```python
from build123d import *

# Parameters (mm, degrees)
PAD_DEPTH       = 35
SKETCH001_W     = 64.566103
SKETCH001_H     = 15
POCKET_DEPTH    = 35
PAD001_DEPTH    = 2
FILLET_R        = 1
FILLET001_R     = 1
FILLET002_R     = 1
FILLET003_R     = 1
FILLET004_R     = 1
PAD002_DEPTH    = 2
FILLET005_R     = 1
FILLET006_R     = 1
FILLET007_R     = 0.8
SKETCH005_R     = 1.8
POCKET001_DEPTH = 5
CHAMFER_SIZE    = 1
CHAMFER001_SIZE = 1
SKETCH006_W     = 10.45074
SKETCH006_H     = 39.185364
POCKET002_DEPTH = 5
SKETCH007_W     = 9.636787
SKETCH007_H     = 41.557176
POCKET003_DEPTH = 5
FILLET008_R     = 10
FILLET009_R     = 10


with BuildPart() as part:
    # Sketch → Pad (new body)
    with BuildSketch(Plane.XY):
        with BuildLine():
            ThreePointArc((25, 0), (0, 25), (-25, 0))
            Line((-27, 0), (-25, 0))
            ThreePointArc((27, 0), (0, 27), (-27, 0))
            Line((27, 0), (25, 0))
        make_face()
    extrude(amount=PAD_DEPTH)

    # Sketch001 (on Face6 of Pad) → Pocket (cut)
    with BuildSketch(Plane.XY.offset(35)):
        with Locations((1.810268, 7.5)):
            Rectangle(SKETCH001_W, SKETCH001_H)
    extrude(amount=-POCKET_DEPTH, mode=Mode.SUBTRACT)

    # Sketch003 (on Face4 of Pocket) → Pad001 (join)
    with BuildSketch(Plane.XY.offset(35)):
        with BuildLine():
            ThreePointArc((25, 15.01), (0, 28.426876), (-25, 15.01))
            Line((-25, -14.99), (-25, 15.01))
            Line((25, -14.99), (-25, -14.99))
            Line((25, 15.01), (25, -14.99))
        make_face()
    extrude(amount=PAD001_DEPTH)

    # Fillet
    fillet_edges = [part.edges().sort_by_distance(p)[0] for p in [
        (25, 0.01, 35),
    ]]
    fillet(fillet_edges, radius=FILLET_R)

    # Fillet001
    fillet001_edges = [part.edges().sort_by_distance(p)[0] for p in [
        (-0.867113, 28.414342, 35),
    ]]
    fillet(fillet001_edges, radius=FILLET001_R)

    # Fillet002
    fillet002_edges = [part.edges().sort_by_distance(p)[0] for p in [
        (-25, -0.933093, 35),
    ]]
    fillet(fillet002_edges, radius=FILLET002_R)

    # Fillet003
    fillet003_edges = [part.edges().sort_by_distance(p)[0] for p in [
        (-22.449944, 15, 17.5),
    ]]
    fillet(fillet003_edges, radius=FILLET003_R)

    # Fillet004
    fillet004_edges = [part.edges().sort_by_distance(p)[0] for p in [
        (22.449944, 15, 17.5),
    ]]
    fillet(fillet004_edges, radius=FILLET004_R)

    # Sketch004 (on Face14 of Fillet004) → Pad002 (join)
    with BuildSketch(Plane(origin=(0, 0, 0), x_dir=(1, 0, 0), z_dir=(0, 0, -1))):
        with BuildLine():
            ThreePointArc((-20, -15), (0.026547, -24.999986), (20.031811, -14.957491))
            Line((20.031811, -14.957491), (24.167366, -17.957491))
            ThreePointArc((-24.136043, -18), (0.026401, -30.182822), (24.167366, -17.957491))
            Line((-20, -15), (-24.136043, -18))
        make_face()
    extrude(amount=PAD002_DEPTH)

    # Fillet005
    fillet005_edges = [part.edges().sort_by_distance(p)[0] for p in [
        (0.026547, 24.999986, -2),
    ]]
    fillet(fillet005_edges, radius=FILLET005_R)

    # Fillet006
    fillet006_edges = [part.edges().sort_by_distance(p)[0] for p in [
        (0.026401, 30.182822, -2),
    ]]
    fillet(fillet006_edges, radius=FILLET006_R)

    # Fillet007
    fillet007_edges = [part.edges().sort_by_distance(p)[0] for p in [
        (0.026401, 30.182822, 0),
    ]]
    fillet(fillet007_edges, radius=FILLET007_R)

    # Sketch005 (on Face18 of Fillet007) → Pocket001 (cut)
    with BuildSketch(Plane(origin=(0, 0, 35), x_dir=(1, 0, 0), z_dir=(0, 0, -1))):
        with Locations((-12.5, 0)):
            Circle(SKETCH005_R)
        with Locations((12.5, 0)):
            Circle(SKETCH005_R)
    extrude(amount=-POCKET001_DEPTH, mode=Mode.SUBTRACT)

    # Chamfer
    chamfer_edges = [part.edges().sort_by_distance(p)[0] for p in [
        (10.7, 0, 35),
    ]]
    chamfer(chamfer_edges, length=CHAMFER_SIZE)

    # Chamfer001
    chamfer001_edges = [part.edges().sort_by_distance(p)[0] for p in [
        (-14.3, 0, 35),
    ]]
    chamfer(chamfer001_edges, length=CHAMFER001_SIZE)

    # Sketch006 (on Face1 of Chamfer001) → Pocket002 (cut)
    with BuildSketch(Plane(origin=(0, 0, 35), x_dir=(1, 0, 0), z_dir=(0, 0, -1))):
        with Locations((-26.72537, -2.508844)):
            Rectangle(SKETCH006_W, SKETCH006_H)
    extrude(amount=-POCKET002_DEPTH, mode=Mode.SUBTRACT)

    # Sketch007 (on Face1 of Pocket002) → Pocket003 (cut)
    with BuildSketch(Plane(origin=(0, 0, 35), x_dir=(1, 0, 0), z_dir=(0, 0, -1))):
        with Locations((26.326259, -1.833993)):
            Rectangle(SKETCH007_W, SKETCH007_H)
    extrude(amount=-POCKET003_DEPTH, mode=Mode.SUBTRACT)

    # Fillet008
    fillet008_edges = [part.edges().sort_by_distance(p)[0] for p in [
        (21.507866, -14.99, 36),
    ]]
    fillet(fillet008_edges, radius=FILLET008_R)

    # Fillet009
    fillet009_edges = [part.edges().sort_by_distance(p)[0] for p in [
        (-21.5, -14.99, 36),
    ]]
    fillet(fillet009_edges, radius=FILLET009_R)


solid = part.part
```
Geometry check sheet. Reference: the model listing, model coordinates, mm. A direction names the side the tool comes from. Coordinates: 2 decimals unless noted, no trailing zeros. Order: outer loops, then holes, each group sorted by start corner. A loop starts at its lowest first (then second) coordinate and runs counter-clockwise, first axis right, second up.
Q1. Depth check by flat-ended pin: pin 1 Ø0.5 at (x, y) = (-20.5, 15.5) entering from -Z; pin 2 Ø12 at (y, z) = (15.5, 25) entering from +X; pin 3 Ø4 at (x, y) = (12.5, 0) entering from -Z; pin 4 Ø3 at (x, y) = (7.5, 12.5) entering from -Z. Enter the tip coordinate at first touch or a pass-through.
Reply:
pin 1: stops at z = -2
pin 2: stops at x = 21.49
pin 3: stops at z = 35.8
pin 4: stops at z = 35
Q2. Draft check along Z on faces 6 (the face through (0, 27, -2)), 7 (the face through (-14.3, -0.08, 36.49)), 8 (the face through (-21.4, 15.58, 17.26)). Enter one of: released by +Z, released by -Z, zero draft, split by the parting line, or undercut.
Reply:
face 6: released by -Z
face 7: zero draft
face 8: undercut
Q3. Tool access check on faces 1 (the face through (21.4, 15.58, 17.26)), 2 (the face through (0.341, 28.425, 36.493)), 3 (the face through (22.071, 16.436, -0.986)), 4 (the face through (-22.04, 16.48, -0.99)), 5 (the face through (0, 27, 17)). Record the directions out of +Z, -Z, +X, -X, +Y, -Y that give a thin tool (end or side, any length) a straight path to the whole face; none if there is none.
Reply:
face 1: +X
face 2: +Z, +Y
face 3: -Z, +X, -Y
face 4: -Z, -X, -Y
face 5: +Y
Q4. Sectioned sample at D-D on y = -12. Record the cut outline in (x, z).
Reply:
outline: (-18.63, 35) - (18.64, 35) - (18.64, 37) - (-18.63, 37) - close
Q5. Sectioned sample at A-A on y = 0. Record the cut outline in (x, z), and give its area (3 significant figures).
Reply:
outline: (-21.5, 35) - (-15.3, 35) - (-14.3, 36) - (-14.3, 37) - (-21.5, 37) - close; (-10.7, 36) - (-9.7, 35) - (9.7, 35) - (10.7, 36) - (10.7, 37) - (-10.7, 37) - close; (14.3, 36) - (15.3, 35) - (21.51, 35) - (21.51, 37) - (14.3, 37) - close
area: 69.6 mm2
Q6. Sectioned sample at C-C on y = 12. Record the cut outline in (x, z).
Reply:
outline: (-21.5, 35) - (21.51, 35) - (21.51, 37) - (-21.5, 37) - close
Q7. Thickness scan on probe 1 along X at (y, z) = (0, 36.8); probe 2 along X at (y, z) = (21, 30.5); probe 3 along Z at (x, y) = (-8.5, 2). Record the ranges inside material, lowest first.
Reply:
probe 1: x = -21.5 to -14.3, -10.7 to 10.7, 14.3 to 21.51
probe 2: x = -16.97 to -13.56, 13.56 to 16.97
probe 3: z = 35 to 37
Q8. Sectioned sample at B-B on z = 4.5. Record the cut outline in (x, y).
Reply:
outline: (-21.28, 16.62) arc R1 ccw to (-20.49, 15) - (-20, 15) arc R25 cw to (20, 15) - (20.49, 15) arc R1 ccw to (21.28, 16.62) arc R27 ccw to start
